from build123d import *

# Parameters (mm, degrees)
SKETCH2_W                             = 29.487
SKETCH2_H                             = 26
BOSS_EXTRUDE1_DEPTH                   = 3.175
CUT_EXTRUDE1_DEPTH                    = 22.900963312
TAP_DRILL_FOR_M3X0_5_TAP1_D           = 2.5
TAP_DRILL_FOR_M3X0_5_TAP1_DEPTH       = 6
TAP_DRILL_FOR_M3X0_5_TAP1_CSINK_D     = 2.55
TAP_DRILL_FOR_M3X0_5_TAP1_CSINK_ANGLE = 90
TAP_DRILL_FOR_M3X0_5_TAP1_TIP         = 0.751075774


with BuildPart() as part:
    # Sketch2 → Boss-Extrude1 (new body)
    with BuildSketch(Plane(origin=(0, 0, 0), x_dir=(0, 1, 0), z_dir=(0, 0, 1))):
        with Locations((-2.5935, 0)):
            Rectangle(SKETCH2_W, SKETCH2_H)
    extrude(amount=BOSS_EXTRUDE1_DEPTH)

    # Sketch1 → Cut-Extrude1 (cut, through all)
    with BuildSketch(Plane(origin=(0, 0, 0), x_dir=(0, 1, 0), z_dir=(0, 0, 1))):
        with BuildLine():
            Line((-9.15, 7.917543811), (-9.15, -7.917543811))
            ThreePointArc((-9.15, -7.917543811), (0, -12.1), (9.15, -7.917543811))
            Line((9.15, -7.917543811), (9.15, 7.917543811))
            ThreePointArc((9.15, 7.917543811), (0, 12.1), (-9.15, 7.917543811))
        make_face()
    extrude(amount=CUT_EXTRUDE1_DEPTH, mode=Mode.SUBTRACT)

    # Tap Drill for M3x0.5 Tap1
    with Locations(Plane(origin=(0, -17.337, 0), x_dir=(-1, 0, 0), z_dir=(0, -1, 0))):
        with Locations((-7.5, -1.5875), (7.5, -1.5875)):
            CounterSinkHole(TAP_DRILL_FOR_M3X0_5_TAP1_D / 2, TAP_DRILL_FOR_M3X0_5_TAP1_CSINK_D / 2, depth=TAP_DRILL_FOR_M3X0_5_TAP1_DEPTH, counter_sink_angle=TAP_DRILL_FOR_M3X0_5_TAP1_CSINK_ANGLE)
            with Locations((0, 0, -(TAP_DRILL_FOR_M3X0_5_TAP1_DEPTH + TAP_DRILL_FOR_M3X0_5_TAP1_TIP / 2))):  # 118° drill point
                Cone(0, TAP_DRILL_FOR_M3X0_5_TAP1_D / 2, TAP_DRILL_FOR_M3X0_5_TAP1_TIP, mode=Mode.SUBTRACT)


solid = part.part
Could you check a few things on this model? Use its own coordinates, in mm. A direction names the side the tool comes from. Give positions to 0.01 mm unless a question says otherwise; leave off trailing zeros. Write each loop counter-clockwise with the first axis right and the second up, starting at its lowest first coordinate (ties: lowest second). Pieces come first, ordered by that corner, then holes. Notation, with made-up numbers: (11, -34) -> (43, -34) arc R22 ccw to (43, -9) -> close; hole circle Ø11 at (3.5, 45). An arc over 180 degrees is marked (long way). Answer as CSV lines item,"result". Start each with the question number.
(1) I'm going to push a flat-ended pin straight in: pin 1 Ø8 at (x, y) = (-3.5, -3.5) entering from +Z. Where does the tip first touch, or does it pass through?
(2) If we mould it in two halves opening along Z, with no side actions, what happens to faces 4 (the face through (0, 12.15, 2)), 5 (the face through (-8.75, -14.28, 1.53)), 6 (the face through (-0.2, -9.4, 0)), 7 (the face through (-0.2, -9.4, 3.175))? For each: +Z half, -Z half, draft (parallel to the pull), parting line (faces both ways), or undercut.
(3) If we section it at A-A, the plane x = -0.75: Write out the boundary of the cut face in (y, z) (3 decimals).
(4) Which directions (+Z, -Z, +X, -X, +Y, -Y) give clear straight access to the entire face, cutting with the end or side of a thin tool? Please do faces 1 (the face through (13, -3, 2)), 2 (the face through (12.1, -0.1, 1.6)), 3 (the face through (6.25, -14.28, 1.53)).
(5) Please list where these lines run through material, in increasing order: line 1 (Y direction, x = 0.75, z = 2.4); line 2 (Z direction, x = -7.5, y = -12.6) (1 decimal); line 3 (X direction, y = -12.75, z = 2).
(6) If we section it at C-C, the plane y = -14.25: Give the number of separate pieces and of enclosed holes in the cut face, and give its area (3 significant figures).
(7) If we section it at B-B, the plane y = -2.25: Write out the boundary of the cut face in (x, z) (3 decimals), and give its area (3 significant figures).
Answer list:
1,pin 1,"through"
2,face 4,"draft"
2,face 5,"undercut"
2,face 6,"-Z half"
2,face 7,"+Z half"
3,outline,"(-17.337, 0) -> (-9.15, 0) -> (-9.15, 3.175) -> (-17.337, 3.175) -> close; (9.15, 0) -> (12.15, 0) -> (12.15, 3.175) -> (9.15, 3.175) -> close"
4,face 1,"+Z, -Z, +X, +Y, -Y"
4,face 2,"+Z, -Z"
4,face 3,"-Y"
5,line 1,"-17.34 to -9.15, 9.15 to 12.15"
5,line 2,"0 to 0.3, 2.8 to 3.2"
5,line 3,"-13 to -8.68, -6.32 to 6.32, 8.68 to 13"
6,separate pieces,"1"
6,enclosed holes,"2"
6,area,"72.7 mm^2"
7,outline,"(-13, 0) -> (-11.889, 0) -> (-11.889, 3.175) -> (-13, 3.175) -> close; (11.889, 0) -> (13, 0) -> (13, 3.175) -> (11.889, 3.175) -> close"
7,area,"7.06 mm^2"
